```python
from build123d import *
from build123d.topology import SkipClean

# Parameters (mm, degrees)
SKETCH1_R        = 7
EXTRUSION1_DEPTH = 7
SKETCH2_R        = 12.5
EXTRUSION2_DEPTH = 53.5
SKETCH3_R        = 3.5
EXTRUSION3_DEPTH = 2.5
EXTRUSION4_DEPTH = 10
SKETCH5_R        = 2
EXTRUSION5_DEPTH = 2
HOLE1_D          = 2
HOLE1_DEPTH      = 10
HOLE1_TIP        = 0.600860619


with BuildPart() as part:
    # Sketch1 → Extrusion1 (new body)
    with BuildSketch(Plane(origin=(0, 0, 0), x_dir=(-1, 0, 0), z_dir=(0, 1, 0))):
        with Locations(Location((0, 0, 0), (0, 0, 90))):
            Circle(SKETCH1_R)
    extrude(amount=EXTRUSION1_DEPTH)

    # Sketch2 → Extrusion2 (add)
    with BuildSketch(Plane(origin=(0, 7, 0), x_dir=(-1, 0, 0), z_dir=(0, 1, 0))):
        with Locations(Location((0, 0, 0), (0, 0, 270))):
            Circle(SKETCH2_R)
    extrude(amount=EXTRUSION2_DEPTH)

    # Sketch3 → Extrusion3 (add)
    with BuildSketch(Plane(origin=(0, 60.5, 0), x_dir=(-1, 0, 0), z_dir=(0, 1, 0))):
        with Locations(Location((0, 0, 0), (0, 0, 90))):
            Circle(SKETCH3_R)
    extrude(amount=EXTRUSION3_DEPTH)

    # Sketch4 → Extrusion4 (add)
    with BuildSketch(Plane(origin=(0, 63, 0), x_dir=(-1, 0, 0), z_dir=(0, 1, 0))):
        with BuildLine():
            Line((1.4, 1.428285686), (1.4, -1.428285686))
            ThreePointArc((1.4, -1.428285686), (-2, 0), (1.4, 1.428285686))
        make_face()
    extrude(amount=EXTRUSION4_DEPTH)

    # Sketch5 → Extrusion5 (add)
    with SkipClean():  # the faces are left unmerged after this step: merging them gives an invalid solid
        with BuildSketch(Plane(origin=(0, 63, 0), x_dir=(1, 0, 0), z_dir=(0, 1, 0))):
            with Locations(Location((0, 0, 0), (0, 0, 134.427004001))):
                Circle(SKETCH5_R)
        extrude(amount=EXTRUSION5_DEPTH)

    # Hole1
    with Locations(Plane(origin=(0, 60.5, 0), x_dir=(1, 0, 0), z_dir=(0, 1, 0))):
        with Locations((0, -9), (0, 9)):
            Hole(HOLE1_D / 2, depth=HOLE1_DEPTH)
            with Locations((0, 0, -(HOLE1_DEPTH + HOLE1_TIP / 2))):  # 118° drill point
                Cone(0, HOLE1_D / 2, HOLE1_TIP, mode=Mode.SUBTRACT)


solid = part.part
```
The listing builds one solid part. Answer for the finished solid, in the listing's coordinates (mm). A direction names the side the tool comes from. Give positions to 0.01 mm unless a question says otherwise; leave off trailing zeros. Order: outer loops, then holes, each group sorted by start corner. A loop starts at its lowest first (then second) coordinate and runs counter-clockwise, first axis right, second up.
1) Determine the mould class of faces 6 (the face through (0, 73, 0)), 7 (the face through (-3.417, 61.732, -0.759)), 8 (the face through (0, 55, -10)) for opening direction Z: pulls with the +Z half, pulls with the -Z half, needs draft (parallel to the pull), parting line crosses it, or undercut.
Reported:
face 6: needs draft
face 7: parting line crosses it
face 8: undercut
2) Find section B-B on y = 58.5. Write down the section's boundary in (x, z), then the cut area to 3 significant figures.
Reported:
outline: circle Ø25 at (0, 0); hole circle Ø2 at (0, -9); hole circle Ø2 at (0, 9)
area: 485 mm2
3) Given P1, Ø3, axis at y = 31.5, z = 2, coming from the -X side; P2, Ø3, axis at x = -3.5, z = -3, coming from the +Y side; P3, Ø3, axis at y = 69, z = 0, coming from the -X side, each flat-ended and moving along its own axis, determine where each tip first touches the part or whether it passes through.
Reported:
P1: stops at x = -12.49
P2: stops at y = 63
P3: stops at x = -1.4
4) Find section C-C on x = -10. Write down the section's boundary in (y, z), then the cut area to 4 significant figures.
Reported:
outline: (7, -7.5) - (60.5, -7.5) - (60.5, 7.5) - (7, 7.5) - close
area: 802.5 mm2
5) Find section D-D on y = 20.5. Write down the section's boundary in (x, z).
Reported:
outline: circle Ø25 at (0, 0)
6) Find section A-A on z = 0. Write down the section's boundary in (x, y).
Reported:
outline: (-12.5, 7) - (-7, 7) - (-7, 0) - (7, 0) - (7, 7) - (12.5, 7) - (12.5, 60.5) - (3.5, 60.5) - (3.5, 63) - (2, 63) - (2, 73) - (-1.4, 73) - (-1.4, 65) - (-2, 65) - (-2, 63) - (-3.5, 63) - (-3.5, 60.5) - (-12.5, 60.5) - close
7) For faces 1 (the face through (-1.4, 69, 0)), 2 (the face through (0, 55, 8)), 3 (the face through (-3.755, 33.376, -11.923)), 4 (the face through (5.4, 7, -5.4)), 5 (the face through (0, 0, 0)), determine the directions among +Z, -Z, +X, -X, +Y, -Y from which every point of the face is accessible in a straight line to the end or side of a thin tool.
Reported:
face 1: +Z, -Z, -X, +Y
face 2: +Y
face 3: +Y, -Y
face 4: -Y
face 5: +Z, -Z, +X, -X, -Y
8) Consider line 1 along Y through (x, z) = (-0.5, 5.75); line 2 along X through (y, z) = (53.5, 9); line 3 along Y through (x, z) = (10, -3.75). Determine where each line is inside the solid, lowest interval first.
Reported:
line 1: y = 0 to 60.5
line 2: x = -8.67 to -1, 1 to 8.67
line 3: y = 7 to 60.5
